Here's the drawing with two shaded views (mm, measured from the low corner). I have some questions. A direction names the side the tool comes from. Round coordinates to 2 decimals unless told otherwise and drop trailing zeros. Loops run counter-clockwise (first coordinate to the right, second up) from the corner with the lowest first, then second, coordinate; pieces in that order, holes last.
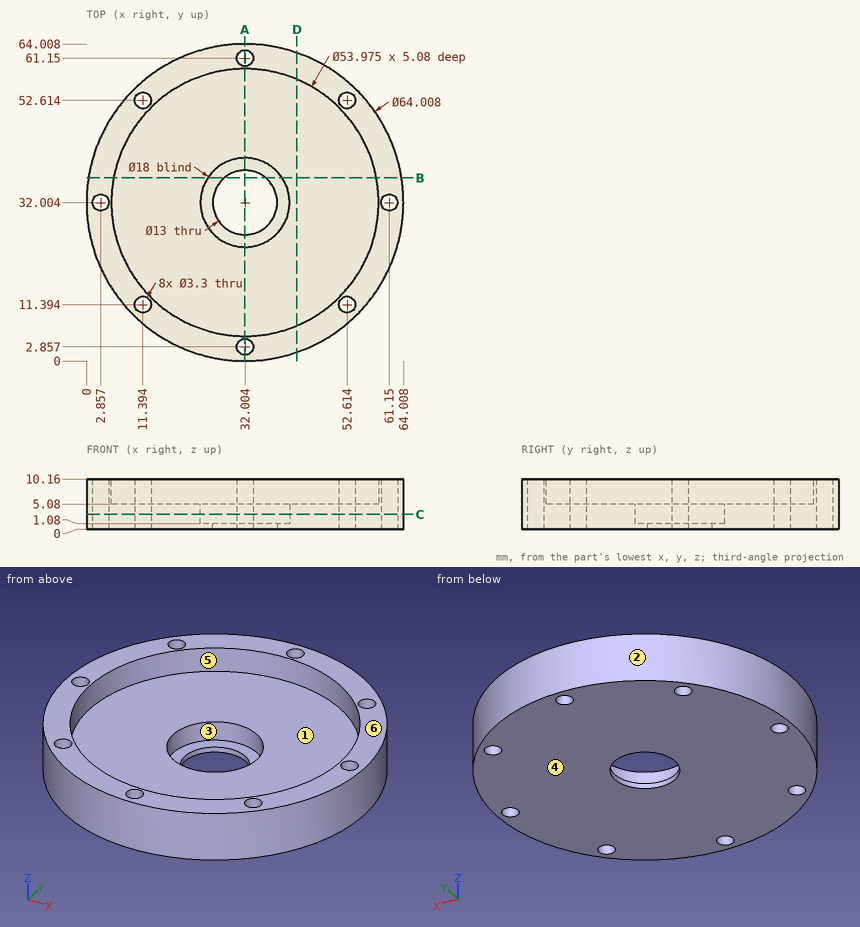
(1) Will these pins go through, and if not, where does the flat tip stop? P1, Ø3, axis at x = 15, z = 8.5, coming from the +Y side; P2, Ø3, axis at x = 13.5, y = 25.5, coming from the -Z side; P3, Ø1.5, axis at y = 37, z = 1.5, coming from the -X side; P4, Ø9, axis at x = 28.5, y = 35.5, coming from the +Z side.
Worked answers:
P1: stops at y = 60
P2: stops at z = 0
P3: stops at x = 0.28
P4: stops at z = 5.08
(2) For the marked faces 5 and 6, which set-ups out of +Z, -Z, +X, -X, +Y, -Y let a thin tool reach every point of the face, with its end or its side?
Worked answers:
face 5: +Z
face 6: +Z, +X, -X, +Y, -Y
(3) If we section it at C-C, the plane z = 3: State how many separate pieces and enclosed holes the cut face has, then the cut area to 4 significant figures.
Worked answers:
separate pieces: 1
enclosed holes: 9
area: 2,895 mm2
(4) If I drill on line 1 (Y direction, x = 33, z = 5.5) (1 decimal); line 2 (Y direction, x = 10, z = 5.75) (1 decimal); line 3 (Z direction, x = 9.5, y = 32.5), over which ranges is the centre line in solid material (lowest first)?
Worked answers:
line 1: y = 0 to 1.5, 4.2 to 5, 59 to 59.8, 62.5 to 64
line 2: y = 8.8 to 10.5, 12.3 to 16.4, 47.6 to 51.7, 53.5 to 55.2
line 3: z = 0 to 5.08
(5) If we mould it in two halves opening along Y, with no side actions, what happens to the marked faces 1, 2, 3 and 4? For each: released by +Y, released by -Y, zero draft, split by the parting line, or undercut.
Worked answers:
face 1: undercut
face 2: split by the parting line
face 3: undercut
face 4: zero draft
(6) If we section it at A-A, the plane x = 32: List the corners of the cut face in (y, z) for me (1 decimal).
Worked answers:
outline: (0, 0) - (1.2, 0) - (1.2, 10.2) - (0, 10.2) - close; (4.5, 0) - (25.5, 0) - (25.5, 1.1) - (23, 1.1) - (23, 5.1) - (5, 5.1) - (5, 10.2) - (4.5, 10.2) - close; (38.5, 0) - (59.5, 0) - (59.5, 10.2) - (59, 10.2) - (59, 5.1) - (41, 5.1) - (41, 1.1) - (38.5, 1.1) - close; (62.8, 0) - (64, 0) - (64, 10.2) - (62.8, 10.2) - close
(7) If we section it at B-B, the plane y = 37: List the corners of the cut face in (x, z) for me (1 decimal).
Worked answers:
outline: (0.4, 0) - (27.8, 0) - (27.8, 1.1) - (24.5, 1.1) - (24.5, 5.1) - (5.5, 5.1) - (5.5, 10.2) - (0.4, 10.2) - close; (36.2, 0) - (63.6, 0) - (63.6, 10.2) - (58.5, 10.2) - (58.5, 5.1) - (39.5, 5.1) - (39.5, 1.1) - (36.2, 1.1) - close
(8) If we section it at D-D, the plane x = 42.5: List the corners of the cut face in (y, z) for me.
Worked answers:
outline: (1.77, 0) - (62.24, 0) - (62.24, 10.16) - (56.87, 10.16) - (56.87, 5.08) - (7.14, 5.08) - (7.14, 10.16) - (1.77, 10.16) - close
